Autodesk Inventor part; units mm, degrees
ref_plane "YZ Plane" through (0, 0, 0) normal (1, 0, 0) x (0, 1, 0)
ref_plane "XZ Plane" through (0, 0, 0) normal (0, 1, 0) x (-1, 0, 0)
ref_plane "XY Plane" through (0, 0, 0) normal (0, 0, 1) x (1, 0, 0)
sketch "Sketch1" plane through (0, 0, 0) normal (0, 1, 0) x (-1, 0, 0)
  line L0 (-10, 10) -> (-10, -10)
  line L1 (-10, -10) -> (10, -10)
  line L2 (10, -10) -> (10, 10)
  line L3 (10, 10) -> (-10, 10)
  line L4 (-10, 10) -> (10, -10) construction
  line L5 (-10, -10) -> (10, 10) construction
  point P0 (0, 0)
  dimension "d0" = 20
  dimension "d1" = 20
extrude "Extrusion1" add sketch "Sketch1" along normal blind 5
sketch "Sketch2" plane through (-10, 0, 10) normal (0, 0, 1) x (1, 0, 0)
  point P0 (10, 0)
sketch "Sketch3" plane through (0, 5, 0) normal (0, 1, 0) x (1, 0, 0)
  point P0 (0, 0)
  point P1 (0, 0)
hole "Hole1" at (0, 5, 0) direction (0, -1, 0) diameter 1.8 end through all counterbore diameter 7.5 counterbore depth 3
sketch "Sketch4" plane through (-10, 0, 10) normal (0, 0, 1) x (1, 0, 0)
  line L0 (10, 0) -> (10, 1.5)
  line L1 (14, 3) -> (14, 0)
  line L2 (14, 0) -> (6, 0)
  line L3 (6, 0) -> (6, 3)
  line L4 (6, 3) -> (14, 3)
  line L5 (14, 3) -> (6, 0) construction
  line L6 (14, 0) -> (6, 3) construction
  dimension "d11" = 8
extrude "Extrusion2" add sketch "Sketch4" along normal blind 8
mirror "Mirror1" about plane through (0, 0, 0) normal (0, 0, 1) of "Extrusion2"
sketch "Sketch5" plane through (0, 5, 0) normal (0, 1, 0) x (1, 0, 0)
  line L0 (0, 0) -> (0, -14)
  line L1 (0, 0) -> (0, 14)
  dimension "d14" = 14
  dimension "d15" = 14
hole "Hole2" at (0, 5, 14) at (0, 5, -14) direction (0, -1, 0) diameter 4.5 end through all
fillet "Fillet1" radius 2 12 edges at (4, 1.5, 10) (4, 1.5, 18) (10, 2.5, 10) (10, 2.5, -10) (4, 1.5, -10) (4, 1.5, -18) (-4, 1.5, -18) (-4, 1.5, -10) (-10, 2.5, -10) (-10, 2.5, 10) (-4, 1.5, 10) (-4, 1.5, 18)
move faces "Move1" translate (0, 2, 0) faces at (0, 3, 10.5833)
move faces "Move2" translate (0, 2, 0) faces at (3.4661, 2, -17.3603) (4.5339, 2, -10.6397) (0, 3, -10.8742)
properties part number "microsoft-lifecam-baseplate"
Here's how the part is built. I have some questions about the finished solid (model axes, mm). A direction names the side the tool comes from. Give positions to 0.01 mm unless a question says otherwise; leave off trailing zeros. Order: outer loops, then holes, each group sorted by start corner. A loop starts at its lowest first (then second) coordinate and runs counter-clockwise, first axis right, second up. Notation, with made-up numbers: (83, -0.5) -> (106, -0.5) arc R12 cw to (106, 3.5) -> close; hole circle Ø4 at (86, 28.5). An arc over 180 degrees is marked (long way). Use a Markdown table: item, result. Add a question column.
Item 1: For faces 1 (the face through (4, 2, -14)), 2 (the face through (4, 3, 14)), 3 (the face through (1, 2, 1)), 4 (the face through (-4, 2, 14)), which set-ups out of +Z, -Z, +X, -X, +Y, -Y let a thin tool reach every point of the face, with its end or its side?
Item 2: Imagine slicing it at D-D on z = 0. Please give me the cut outline in (x, y), plus the area to 3 significant figures.
Item 3: Imagine slicing it at B-B on y = 1.05. Please give me the cut outline in (x, z).
Item 4: If we mould it in two halves opening along Z, with no side actions, what happens to faces 5 (the face through (4.57, 2.46, 10.6)), 6 (the face through (10, 2, 0)), 7 (the face through (-0.676, 2.465, 16.146))? For each: pulls with the +Z half, pulls with the -Z half, needs draft (parallel to the pull), parting line crosses it, or undercut.
Item 5: Will these pins go through, and if not, where does the flat tip stop? pin 1 (1.6 mm diameter, centred on x = 0, z = 0, fed in from +Y); pin 2 (3 mm diameter, centred on y = 1.5, z = -15, fed in from -X); pin 3 (0.6 mm diameter, centred on x = -7, y = 3, fed in from -Z); pin 4 (1.6 mm diameter, centred on x = -7.5, y = 1.5, fed in from +Z).
Item 6: Imagine slicing it at A-A on z = 14. Please give me the cut outline in (x, y), plus the area to 3 significant figures.
Item 7: I need wall thicknesses on line 1 (Z direction, x = 0, y = 1.4); line 2 (Z direction, x = 0, y = 2.95); line 3 (X direction, y = 3.3, z = -14). Which ranges of each line are inside material? Lowest first, please.
Item 8: Imagine slicing it at C-C on x = 0. Please give me the cut outline in (y, z), plus the area to 3 significant figures.
Data:
| question | item | result |
|---|---|---|
| 1 | face 1 | -Z, +X, +Y, -Y |
| 1 | face 2 | +Z, +X, +Y, -Y |
| 1 | face 3 | +Y |
| 1 | face 4 | +Z, -X, +Y, -Y |
| 2 | outline | (-10, 0) -> (-0.9, 0) -> (-0.9, 2) -> (-3.75, 2) -> (-3.75, 5) -> (-10, 5) -> close; (0.9, 0) -> (10, 0) -> (10, 5) -> (3.75, 5) -> (3.75, 2) -> (0.9, 2) -> close |
| 2 | area | 73.9 mm² |
| 3 | outline | (-10, -8) arc R2 ccw to (-8, -10) -> (-6, -10) arc R2 cw to (-4, -12) -> (-4, -16) arc R2 ccw to (-2, -18) -> (2, -18) arc R2 ccw to (4, -16) -> (4, -12) arc R2 cw to (6, -10) -> (8, -10) arc R2 ccw to (10, -8) -> (10, 8) arc R2 ccw to (8, 10) -> (6, 10) arc R2 cw to (4, 12) -> (4, 16) arc R2 ccw to (2, 18) -> (-2, 18) arc R2 ccw to (-4, 16) -> (-4, 12) arc R2 cw to (-6, 10) -> (-8, 10) arc R2 ccw to (-10, 8) -> close; hole circle Ø4.5 at (0, -14); hole circle Ø4.5 at (0, 14); hole circle Ø1.8 at (0, 0) |
| 4 | face 5 | pulls with the +Z half |
| 4 | face 6 | needs draft |
| 4 | face 7 | undercut |
| 5 | pin 1 | passes through |
| 5 | pin 2 | stops at x = -4 |
| 5 | pin 3 | stops at z = -10 |
| 5 | pin 4 | stops at z = 10 |
| 6 | outline | (-4, 0) -> (-2.25, 0) -> (-2.25, 5) -> (-4, 5) -> close; (2.25, 0) -> (4, 0) -> (4, 5) -> (2.25, 5) -> close |
| 6 | area | 17.5 mm² |
| 7 | line 1 | z = -18 to -16.25, -11.75 to -0.9, 0.9 to 11.75, 16.25 to 18 |
| 7 | line 2 | z = -18 to -16.25, -11.75 to -3.75, 3.75 to 11.75, 16.25 to 18 |
| 7 | line 3 | x = -4 to -2.25, 2.25 to 4 |
| 8 | outline | (0, -18) -> (5, -18) -> (5, -16.25) -> (0, -16.25) -> close; (0, -11.75) -> (5, -11.75) -> (5, -3.75) -> (2, -3.75) -> (2, -0.9) -> (0, -0.9) -> close; (0, 0.9) -> (2, 0.9) -> (2, 3.75) -> (5, 3.75) -> (5, 11.75) -> (0, 11.75) -> close; (0, 16.25) -> (5, 16.25) -> (5, 18) -> (0, 18) -> close |
| 8 | area | 109 mm² |
